from build123d import *

# Parameters (mm, degrees)
SKETCH1_R           = 8
BOSS_EXTRUDE1_DEPTH = 600
CHAMFER1_SIZE       = 1


with BuildPart() as part:
    # Sketch1 → Boss-Extrude1 (new, symmetric)
    with BuildSketch(Plane.XY):
        Circle(SKETCH1_R)
    extrude(amount=BOSS_EXTRUDE1_DEPTH, both=True)

    # Sketch4 → CSK for M2.5 Flat Head Machine Screw1 (revolve, cut)
    with BuildSketch(Plane(origin=(0, 0, -600), x_dir=(0, 1, 0), z_dir=(1, 0, 0))):
        Polygon((0, 0), (0, 5), (1.45, 4.128752102), (1.45, 2.25166605), (2.75, 0), align=None)
    csk_for_m2_5_flat_head_machine_screw1 = revolve(axis=Axis((0, 0, -606.35), (0, 0, 1)), mode=Mode.SUBTRACT)

    # Mirror1: CSK for M2.5 Flat Head Machine Screw1 across plane
    add(csk_for_m2_5_flat_head_machine_screw1.mirror(Plane.XY), mode=Mode.SUBTRACT)

    # Chamfer1
    chamfer1_edges = [part.edges().sort_by_distance(p)[0] for p in [
        (-8, 0, -600),
        (-8, 0, 600),
    ]]
    chamfer(chamfer1_edges, length=CHAMFER1_SIZE)


solid = part.part
Design review of the part built by this model. Coordinates are the model's own, in mm. Coordinates: 2 decimals unless noted, no trailing zeros. Order: outer loops, then holes, each group sorted by start corner. A loop starts at its lowest first (then second) coordinate and runs counter-clockwise, first axis right, second up.
Item 1: For pin 1 Ø3 at (x, z) = (-4, 470) entering from -Y; pin 2 Ø4.5 at (x, y) = (0, 0) entering from +Z; pin 3 Ø1.5 at (y, z) = (-6, 109) entering from -X, all flat-tipped, find the tip position at first contact; note any pin that passes through.
Item 2: For line 1 (Y direction, x = 0, z = -596.3); line 2 (Y direction, x = -1, z = -189); line 3 (Z direction, x = 2.25, y = 0.5), list the stretches that pass through material, from the lowest coordinate up.
Item 3: Take a section at A-A, the plane z = 0.5. Write out the cut boundary in (x, y).
The answers:
1. pin 1: stops at y = -7.6
1. pin 2: stops at z = 599.13
1. pin 3: stops at x = -6.04
2. line 1: y = -8 to -1.45, 1.45 to 8
2. line 2: y = -7.94 to 7.94
2. line 3: z = -599.23 to 599.23
3. outline: circle Ø16 at (0, 0)
